from build123d import *

# Parameters (mm, degrees)
PAD_DEPTH    = 20
FILLET_R     = 11
FILLET001_R  = 10
THICKNESS_T  = -1.5
SKETCH001_W  = 1.5
SKETCH001_H  = 20
PAD001_DEPTH = 6


with BuildPart() as part:
    # Sketch → Pad (new body)
    with BuildSketch(Plane.XY):
        Polygon((0, 0), (18, 0), (18, -10), (-7.514719, -18), (-16, -15), (0, -8), align=None)
    extrude(amount=PAD_DEPTH)

    # Fillet
    fillet_edges = [part.edges().sort_by_distance(p)[0] for p in [
        (18, -10, 10),
    ]]
    fillet(fillet_edges, radius=FILLET_R)

    # Fillet001
    fillet001_edges = [part.edges().sort_by_distance(p)[0] for p in [
        (0, -8, 10),
    ]]
    fillet(fillet001_edges, radius=FILLET001_R)

    # Thickness
    thickness_openings = [part.faces().sort_by_distance(p)[0] for p in [
        (9, 0, 10),
        (-11.757359, -16.5, 10),
    ]]
    offset(amount=THICKNESS_T, openings=thickness_openings)

    # Sketch001 → Pad001 (new body)
    with BuildSketch(Plane(origin=(0, 0, 0), x_dir=(-1, 0, 0), z_dir=(0, 1, 0))):
        with Locations((-17.25, 10)):
            Rectangle(SKETCH001_W, SKETCH001_H)
        with Locations((-0.75, 10)):
            Rectangle(SKETCH001_W, SKETCH001_H)
    extrude(amount=PAD001_DEPTH)


solid = part.part
Can you work these out from the model? Positions are in its coordinate system, mm. A direction names the side the tool comes from. Round coordinates to 2 decimals unless told otherwise and drop trailing zeros. Write each loop counter-clockwise with the first axis right and the second up, starting at its lowest first coordinate (ties: lowest second). Pieces come first, ordered by that corner, then holes. Notation, with made-up numbers: (-22, 47) - (-7, 47) arc R18 ccw to (-7, 67) - close; hole circle Ø9 at (64, 51). An arc over 180 degrees is marked (long way). Write each question's results on one line, items separated by ' | '. Start each with the question number.
1) Suppose I cut it at A-A (z = 15.75). List the corners of the cut face in (x, y) for me, and give its area (3 significant figures).
2) Suppose I cut it at C-C (x = 0.5). List the corners of the cut face in (y, z) for me.
3) Which directions (+Z, -Z, +X, -X, +Y, -Y) give clear straight access to the entire face, cutting with the end or side of a thin tool? Please do faces 1 (the cylindrical face through (-0.325, -7.676, 10.119)), 2 (the flat face through (9, 0, 1)), 3 (the flat face through (0, 2, 10)).
4) For pin 1 Ø5 at (x, z) = (6, 8) entering from +Y; pin 2 Ø0.8 at (x, z) = (8, 0.5) entering from +Y; pin 3 Ø5 at (y, z) = (-6.5, 6) entering from -X, each with a flat end and sliding along its axis, tell me the tip position at first contact or that it passes through.
5) Please list where these lines run through material, in increasing order: line 1 (X direction, y = 2.75, z = 8.25); line 2 (Z direction, x = 14, y = -7.5); line 3 (X direction, y = -5.5, z = 8.5).
6) Suppose I cut it at B-B (y = 3.25). List the corners of the cut face in (x, z) for me.
7) Suppose I cut it at D-D (y = -14.25). List the corners of the cut face in (x, z) for me, and give its area (3 significant figures).
8) We'd pull the mould along Y, two halves only. Please class faces 4 (the flat face through (1, 6, 10)), 5 (the flat face through (0.124, -14.033, 9.881)), 6 (the flat face through (16.5, 2, 10)): released by +Y, released by -Y, zero draft, split by the parting line, or undercut.
Here are the results:
1) outline: (-16, -15) - (-13.93, -15.73) - (-5.39, -12) arc R11.5 ccw to (1.5, -1.46) - (1.5, 6) - (0, 6) - (0, -1.46) arc R10 cw to (-5.99, -10.62) - close; (-9.87, -17.17) - (-7.51, -18) - (10.29, -12.42) arc R11 ccw to (18, -1.92) - (18, 6) - (16.5, 6) - (16.5, -1.92) arc R9.5 cw to (9.84, -10.99) - close | area: 106 mm2
2) outline: (-15.49, 0) - (6, 0) - (6, 20) - (-15.49, 20) - close; hole (-13.92, 1.5) - (-6.15, 1.5) - (-6.15, 18.5) - (-13.92, 18.5) - close
3) face 1: none | face 2: +Z, -Z, +Y | face 3: +Z, -Z, -X, +Y
4) pin 1: stops at y = -11.41 | pin 2: stops at y = 0 | pin 3: stops at x = -3.43
5) line 1: x = 0 to 1.5, 16.5 to 18 | line 2: z = 0 to 1.5, 18.5 to 20 | line 3: x = -0.85 to 0.77, 15.8 to 17.4
6) outline: (0, 0) - (1.5, 0) - (1.5, 20) - (0, 20) - close; (16.5, 0) - (18, 0) - (18, 20) - (16.5, 20) - close
7) outline: (-14.29, 0) - (4.45, 0) - (4.45, 20) - (-14.29, 20) - close; hole (-10.54, 1.5) - (-0.57, 1.5) - (-0.57, 18.5) - (-10.54, 18.5) - close | area: 205 mm2
8) face 4: released by +Y | face 5: undercut | face 6: zero draft
